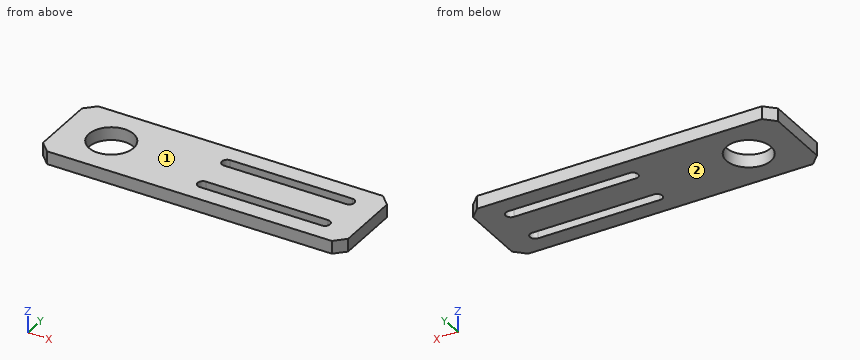
```python
from build123d import *

# Parameters (mm, degrees)
SKETCH1_W           = 205
SKETCH1_H           = 42
BOSS_EXTRUDE1_DEPTH = 6.35
SKETCH4_R           = 11
CUT_EXTRUDE3_DEPTH  = 7.35
CHAMFER1_SIZE       = 5
SKETCH9_R           = 11
CUT_EXTRUDE8_DEPTH  = 7.35
SKETCH13_R          = 11
CUT_EXTRUDE10_DEPTH = 10


with BuildPart() as part:
    # Sketch1 → Boss-Extrude1 (new body)
    with BuildSketch(Plane.XY):
        Rectangle(SKETCH1_W, SKETCH1_H)
    extrude(amount=BOSS_EXTRUDE1_DEPTH)

    # Sketch4 → Cut-Extrude3 (cut, through all)
    with BuildSketch(Plane.XY.offset(6.35)):
        with Locations((-78.5, 0)):
            Circle(SKETCH4_R)
    extrude(amount=-CUT_EXTRUDE3_DEPTH, mode=Mode.SUBTRACT)

    # Chamfer1
    chamfer1_edges = [part.edges().sort_by_distance(p)[0] for p in [
        (102.5, -21, 3.175),
        (-102.5, -21, 3.175),
        (-102.5, 21, 3.175),
        (102.5, 21, 3.175),
    ]]
    chamfer(chamfer1_edges, length=CHAMFER1_SIZE)

    # Sketch9 → Cut-Extrude8 (cut, through all)
    with BuildSketch(Plane.XY.offset(6.35)):
        with Locations((82.5, 0)):
            Circle(SKETCH9_R)
    extrude(amount=-CUT_EXTRUDE8_DEPTH, mode=Mode.SUBTRACT)

    # Sketch13 → Cut-Extrude10 (cut)
    with BuildSketch(Plane.XY.offset(6.35)):
        Polygon((42.5, 21), (47.5, 16), (47.5, -16), (42.5, -21), (97.5, -21), (102.5, -16), (102.5, 16), (97.5, 21), align=None)
        with Locations((82.5, 0)):
            Circle(SKETCH13_R, mode=Mode.SUBTRACT)
        with BuildLine():
            Line((-27.5, 7.46), (32.5, 7.46))
            ThreePointArc((32.5, 7.46), (35.04, 10), (32.5, 12.54))
            Line((32.5, 12.54), (-27.5, 12.54))
            ThreePointArc((-27.5, 12.54), (-30.04, 10), (-27.5, 7.46))
        make_face()
        with BuildLine():
            ThreePointArc((32.5, -7.46), (35.04, -10), (32.5, -12.54))
            Line((32.5, -12.54), (-27.5, -12.54))
            ThreePointArc((-27.5, -12.54), (-30.04, -10), (-27.5, -7.46))
            Line((-27.5, -7.46), (32.5, -7.46))
        make_face()
    extrude(amount=-CUT_EXTRUDE10_DEPTH, mode=Mode.SUBTRACT)


solid = part.part
```
Geometry: final body of the model. Coordinates: model frame, mm. Face numbers are marked on the shaded views. Coordinates: 2 decimals unless noted, no trailing zeros. Order: outer loops, then holes, each group sorted by start corner. A loop starts at its lowest first (then second) coordinate and runs counter-clockwise, first axis right, second up. Notation, with made-up numbers: M 75.25,24 L 106.25,24 A11 cw 106.25,34 Z; hole C 49,39.5 d10. An arc over 180 degrees is marked long. Answer in a Markdown table with one row per item. Add a question column.
Q1. Section query B-B on y = 4. Return the cut outline in (x, z), and give its area (3 significant figures).
Q2. Section query D-D on x = -78.5. Return the cut outline in (y, z), and give its area (3 significant figures).
Q3. Line query: L1, parallel to Y at x = -5, z = 0.5; L2, parallel to Y at x = -78.5, z = 4; L3, parallel to X at y = -10, z = 4. Output: solid intervals per line, ascending.
Q4. Section query A-A on x = 28.5. Return the cut outline in (y, z), and give its area (3 significant figures).
Q5. Mould query, pull axis Z, two halves, no side actions, for the marked faces 1 and 2. Classes: released by +Z, released by -Z, zero draft, split by the parting line, or undercut.
Q6. Contact query for a flat-ended pin moving along its axis: P1, Ø2, axis at x = 28.5, y = -10.5, coming from the -Z side. Output: stop coordinate, or through.
Q7. Section query C-C on z = 2.25. Return the cut outline in (x, y), and give its area (3 significant figures).
Completed:
| question | item | result |
|---|---|---|
| 1 | outline | M -102.5,0 L -88.75,0 L -88.75,6.35 L -102.5,6.35 Z; M -68.25,0 L 47.5,0 L 47.5,6.35 L -68.25,6.35 Z |
| 1 | area | 822 mm2 |
| 2 | outline | M -21,0 L -11,0 L -11,6.35 L -21,6.35 Z; M 11,0 L 21,0 L 21,6.35 L 11,6.35 Z |
| 2 | area | 127 mm2 |
| 3 | L1 | y = -21 to -12.54, -7.46 to 7.46, 12.54 to 21 |
| 3 | L2 | y = -21 to -11, 11 to 21 |
| 3 | L3 | x = -102.5 to -83.08, -73.92 to -30.04, 35.04 to 47.5 |
| 4 | outline | M -21,0 L -12.54,0 L -12.54,6.35 L -21,6.35 Z; M -7.46,0 L 7.46,0 L 7.46,6.35 L -7.46,6.35 Z; M 12.54,0 L 21,0 L 21,6.35 L 12.54,6.35 Z |
| 4 | area | 202 mm2 |
| 5 | face 1 | released by +Z |
| 5 | face 2 | released by -Z |
| 6 | P1 | passes through |
| 7 | outline | M -102.5,-16 L -97.5,-21 L 42.5,-21 L 47.5,-16 L 47.5,16 L 42.5,21 L -97.5,21 L -102.5,16 Z; hole C -78.5,0 d22; hole M -27.5,-12.54 L 32.5,-12.54 A2.54 ccw 32.5,-7.46 L -27.5,-7.46 A2.54 ccw Z; hole M -27.5,7.46 L 32.5,7.46 A2.54 ccw 32.5,12.54 L -27.5,12.54 A2.54 ccw Z |
| 7 | area | 5,220 mm2 |
